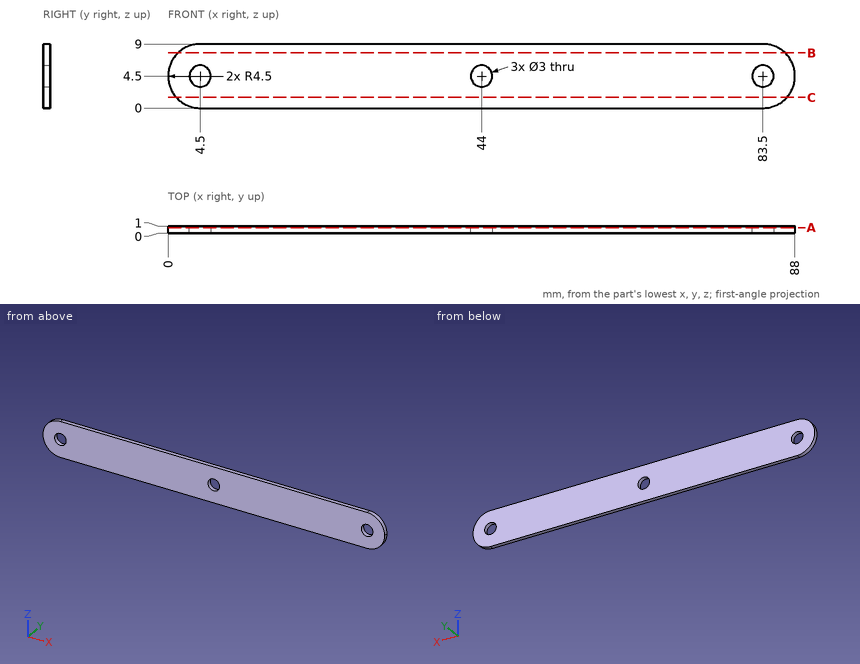
For this review, use the dimensioned drawing (mm, ordinates from the lowest corner) and the shaded views. Coordinates: 2 decimals unless noted, no trailing zeros. Write each loop counter-clockwise with the first axis right and the second up, starting at its lowest first coordinate (ties: lowest second). Pieces come first, ordered by that corner, then holes. Notation, with made-up numbers: (-32.5, -18) - (-25.5, -18) arc R14 cw to (-25.5, 1) - close; hole circle Ø8 at (-28, 89). An arc over 180 degrees is marked (long way). Answer in a Markdown table with one row per item. Add a question column.
Q1. Clearance check with a flat-ended pin moving along its axis: pin 1 (5 mm diameter, centred on x = 83.5, z = 4.5, fed in from +Y). State where the tip first meets the part, or that it passes through.
Q2. To check wall thickness, follow line 1 along Z through (x, y) = (44, 0.2); line 2 along X through (y, z) = (0.9, 5.75); line 3 along X through (y, z) = (0.35, 5.5). State the ranges of each line that lie inside material, in increasing order. Write a range as from..to.
Q3. Consider section B-B on z = 7.75. Give the boundary of the cut face in (x, y), then the cut area to 3 significant figures.
Q4. Consider section A-A on y = 0.8. Give the boundary of the cut face in (x, z).
Q5. Consider section C-C on z = 1.5. Give the boundary of the cut face in (x, y), then the cut area to 3 significant figures.
Answers below:
| question | item | result |
|---|---|---|
| 1 | pin 1 | y = 1 |
| 2 | line 1 | 0..3, 6..9 |
| 2 | line 2 | 0.18..3.67, 5.33..43.17, 44.83..82.67, 84.33..87.82 |
| 2 | line 3 | 0.11..3.38, 5.62..42.88, 45.12..82.38, 84.62..87.89 |
| 3 | outline | (1.39, 0) - (86.61, 0) - (86.61, 1) - (1.39, 1) - close |
| 3 | area | 85.2 mm² |
| 4 | outline | (4.5, 0) - (83.5, 0) arc R4.5 ccw to (88, 4.5) arc R4.5 ccw to (83.5, 9) - (4.5, 9) arc R4.5 ccw to start; hole circle Ø3 at (4.5, 4.5); hole circle Ø3 at (44, 4.5); hole circle Ø3 at (83.5, 4.5) |
| 5 | outline | (1.15, 0) - (86.85, 0) - (86.85, 1) - (1.15, 1) - close |
| 5 | area | 85.7 mm² |
